For this review, take the finished solid that the model builds, in its own axes (mm). Face numbers are marked on the shaded views. A direction names the side the tool comes from. Round coordinates to 2 decimals unless told otherwise and drop trailing zeros. Order: outer loops, then holes, each group sorted by start corner. A loop starts at its lowest first (then second) coordinate and runs counter-clockwise, first axis right, second up. Notation, with made-up numbers: (83.25, 65.25) -> (132.25, 65.25) arc R23 ccw to (132.25, 85.25) -> close; hole circle Ø1 at (87.25, 5). An arc over 180 degrees is marked (long way). Use a Markdown table: item, result. Add a question column.
1) Draft analysis for pull direction Y (two halves, no side actions). For the marked faces 1, 2 and 3, state which applies: pulls with the +Y half, pulls with the -Y half, needs draft (parallel to the pull), parting line crosses it, or undercut.
2) Machinability: for the marked faces 4 and 5, which of the approach directions +Z, -Z, +X, -X, +Y, -Y give a long, thin tool a straight path to every point of the face, cutting with its end or side? Answer none if there is none.
3) Consider section A-A (z = 14). State the section outline as (x, y) points, plus the area to 3 significant figures.
4) Consider section C-C (x = 30.5). State the section outline as (y, z) points.
5) Wall thickness on line 1 along Y through (x, z) = (36.75, 30); line 2 along X through (y, z) = (-1, 29); line 3 along Y through (x, z) = (-37, 17.5): over which ranges is each line inside the solid? List them lowest first. Write a range as [from, to].
6) Consider section B-B (y = 25.5). State the section outline as (x, z) points.
7) Clearance check with flat-ended pins moving along their axes: P1, Ø2, axis at x = -37, y = -0.5, coming from the -Z side; P2, Ø1.6, axis at y = -21, z = 5, coming from the +X side; P3, Ø3.5, axis at y = -36, z = 30, coming from the -X side; P4, Ø1.6, axis at y = -36, z = 30, coming from the -X side. State where each tip first meets the part, or that it passes through.
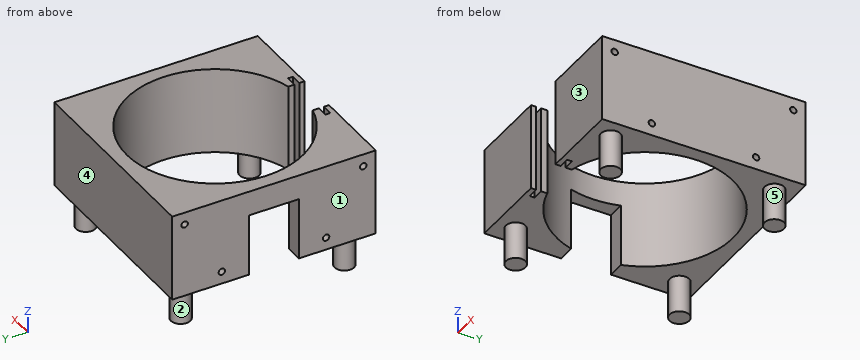
```python
from build123d import *

# Parameters (mm, degrees)
SKETCH_1_W               = 82
SKETCH_1_H               = 82
SKETCH_1_R               = 35.5
EXTRUDE_1_DEPTH          = 35
CUT_EXTRUDE_1_REACH      = 79.727
CUT_EXTRUDE_START        = -10
SKETCH_2_W               = 8
SKETCH_2_H               = 20
SKETCH_3_R               = 3.95
EXTRUDE_2_DEPTH          = 15
PATTERN_CIRCULAR_1_COUNT = 4
SKETCH_4_R               = 1.3
CUT_EXTRUDE_2_DEPTH      = 9
MIRROR_4_COPY_1_SKETCH_R = 1.3
MIRROR_4_COPY_1_DEPTH    = 9
CUT_EXTRUDE_3_DEPTH      = 77.56369897


with BuildPart() as part:
    # Sketch 1 → Extrude 1 (new body)
    with BuildSketch(Plane.XY):
        Rectangle(SKETCH_1_W, SKETCH_1_H)
        Circle(SKETCH_1_R, mode=Mode.SUBTRACT)
    extrude(amount=EXTRUDE_1_DEPTH)

    # Sketch 2 → Cut-Extrude 1 (cut, up to next)
    with BuildSketch(Plane.XY.offset(35).offset(CUT_EXTRUDE_START), mode=Mode.PRIVATE) as cut_extrude_1_sk1:
        with Locations((-37, 0)):
            Rectangle(SKETCH_2_W, SKETCH_2_H)
    cut_extrude_1_tool1 = extrude(cut_extrude_1_sk1.sketch, amount=-CUT_EXTRUDE_1_REACH, mode=Mode.PRIVATE) & part.part
    add(cut_extrude_1_tool1.solids().sort_by_distance((-37, 0, 25))[0], mode=Mode.SUBTRACT)

    # Sketch 3 → Extrude 2 (add)
    with BuildSketch(Plane(origin=(0, 0, 0), x_dir=(-1, 0, 0), z_dir=(0, 0, -1))):
        with Locations((33, 33)):
            Circle(SKETCH_3_R)
    extrude_2 = extrude(amount=EXTRUDE_2_DEPTH)

    # Pattern Circular 1: Extrude 2 ×4 about axis
    pattern_circular_1_axis = Axis((0, 0, 0), (0, 0, 1))
    for i in range(1, PATTERN_CIRCULAR_1_COUNT):
        add(extrude_2.rotate(pattern_circular_1_axis, i * 360 / PATTERN_CIRCULAR_1_COUNT))

    # Sketch 4 → Cut-Extrude 2 (cut)
    with BuildSketch(Plane.ZY.offset(41)):
        with Locations((5, -21)):
            Circle(SKETCH_4_R)
        with Locations((30, -36)):
            Circle(SKETCH_4_R)
    cut_extrude_2 = extrude(amount=-CUT_EXTRUDE_2_DEPTH, mode=Mode.SUBTRACT)

    # Mirror 2: Cut-Extrude 2 across plane
    add(cut_extrude_2.mirror(Plane.ZX), mode=Mode.SUBTRACT)

    # Mirror 4: Cut-Extrude 2 across plane
    add(cut_extrude_2.mirror(Plane(origin=(0, 0, 0), x_dir=(0, 0, 1), z_dir=(1, 0, 0))), mode=Mode.SUBTRACT)

    # Mirror 4 copy 1 sketch → Mirror 4 copy 1 (cut)
    with BuildSketch(Plane(origin=(41, 0, 0), x_dir=(0, 0, 1), z_dir=(1, 0, 0))):
        with Locations((5, -21)):
            Circle(MIRROR_4_COPY_1_SKETCH_R)
        with Locations((30, -36)):
            Circle(MIRROR_4_COPY_1_SKETCH_R)
    extrude(amount=-MIRROR_4_COPY_1_DEPTH, mode=Mode.SUBTRACT)

    # Sketch 5 → Cut-Extrude 3 (cut, through all)
    with BuildSketch(Plane.XY.offset(35)):
        Polygon((-8.5, -36.967375879), (-8.5, -34.467375879), (8.5, -34.467375879), (8.5, -36.967375879), (13, -36.967375879), (13, -38.967375879), (8.5, -38.967375879), (8.5, -41.467375879), (-8.5, -41.467375879), (-8.5, -38.967375879), (-13, -38.967375879), (-13, -36.967375879), align=None)
    extrude(amount=-CUT_EXTRUDE_3_DEPTH, mode=Mode.SUBTRACT)


solid = part.part
```
Results list:
| question | item | result |
|---|---|---|
| 1 | face 1 | needs draft |
| 1 | face 2 | undercut |
| 1 | face 3 | pulls with the -Y half |
| 2 | face 4 | +Z, -Z, +X, -X, +Y |
| 2 | face 5 | -Z |
| 3 | outline | (-41, -41) -> (-8.5, -41) -> (-8.5, -38.97) -> (-13, -38.97) -> (-13, -36.97) -> (-8.5, -36.97) -> (-8.5, -34.47) arc R35.5 cw to (-34.06, -10) -> (-41, -10) -> close; (-41, 10) -> (-34.06, 10) arc R35.5 cw (long way) to (8.5, -34.47) -> (8.5, -36.97) -> (13, -36.97) -> (13, -38.97) -> (8.5, -38.97) -> (8.5, -41) -> (41, -41) -> (41, 41) -> (-41, 41) -> close |
| 3 | area | 2,530 mm2 |
| 4 | outline | (-41, 0) -> (-36.06, 0) -> (-36.06, -15) -> (-29.94, -15) -> (-29.94, 0) -> (-18.17, 0) -> (-18.17, 35) -> (-41, 35) -> close; (18.17, 0) -> (29.94, 0) -> (29.94, -15) -> (36.06, -15) -> (36.06, 0) -> (41, 0) -> (41, 35) -> (18.17, 35) -> close |
| 5 | line 1 | [-41, -37.3], [-34.7, 34.7], [37.3, 41] |
| 5 | line 2 | [-41, -35.49], [35.49, 41] |
| 5 | line 3 | [-41, -10], [10, 41] |
| 6 | outline | (-41, 0) -> (-24.7, 0) -> (-24.7, 35) -> (-41, 35) -> close; (24.7, 0) -> (41, 0) -> (41, 35) -> (24.7, 35) -> close |
| 7 | P1 | z = 25 |
| 7 | P2 | x = 32 |
| 7 | P3 | x = -41 |
| 7 | P4 | x = -32 |
